```python
from build123d import *

# Parameters (mm, degrees)
SKETCH1_R           = 20
BOSS_EXTRUDE1_DEPTH = 10
SKETCH2_R           = 25
BOSS_EXTRUDE2_DEPTH = 60
FILLET1_R           = 25
SKETCH3_W           = 23.240720894
SKETCH3_H           = 7.34315937
BOSS_EXTRUDE3_DEPTH = 120
SKETCH4_R           = 7.943437771
BOSS_EXTRUDE4_DEPTH = 60
FILLET2_R           = 7
FILLET3_R           = 7
FILLET4_SIZE        = 10
FILLET4_SIZE_2      = 13


with BuildPart() as part:
    # Sketch1 → Boss-Extrude1 (new body)
    with BuildSketch(Plane(origin=(0, 0, 0), x_dir=(0, 0, -1), z_dir=(1, 0, 0))):
        Circle(SKETCH1_R)
    extrude(amount=BOSS_EXTRUDE1_DEPTH)

    # Sketch2 → Boss-Extrude2 (add)
    with BuildSketch(Plane(origin=(10, 0, 0), x_dir=(0, 0, -1), z_dir=(1, 0, 0))):
        Circle(SKETCH2_R)
    extrude(amount=BOSS_EXTRUDE2_DEPTH)

    # Fillet1
    fillet1_edges = [part.edges().sort_by_distance(p)[0] for p in [
        (70, 0, 25),
    ]]
    fillet(fillet1_edges, radius=FILLET1_R)

    # Sketch3 → Boss-Extrude3 (add)
    with BuildSketch(Plane.ZY):
        Rectangle(SKETCH3_W, SKETCH3_H)
    extrude(amount=-BOSS_EXTRUDE3_DEPTH)

    # Sketch4 → Boss-Extrude4 (add, symmetric)
    with BuildSketch(Plane(origin=(0, 3.671579685, 0), x_dir=(1, 0, 0), z_dir=(0, 1, 0))):
        with Locations(Location((103.030776269, 0, 0), (0, 0, 270))):
            Circle(SKETCH4_R)
    extrude(amount=BOSS_EXTRUDE4_DEPTH, both=True)

    # Fillet2
    fillet2_edges = [part.edges().sort_by_distance(p)[0] for p in [
        (103.030776269, 63.671579685, -7.943437771),
    ]]
    fillet(fillet2_edges, radius=FILLET2_R)

    # Fillet3
    fillet3_edges = [part.edges().sort_by_distance(p)[0] for p in [
        (103.030776269, -56.328420315, -7.943437771),
    ]]
    fillet(fillet3_edges, radius=FILLET3_R)

    # Fillet4
    # an asymmetric fillet: 13, 10 mm, written as the material it takes off along each edge
    with BuildSketch(Plane(origin=(120, -36.171579685, -11.620360447), x_dir=(-1, 0, 0), z_dir=(0, 1, 0)), Plane(origin=(120, 36.171579685, 11.620360447), x_dir=(-1, 0, 0), z_dir=(0, -1, 0))) as fillet4_piece_1:
        with BuildLine():
            Bezier((FILLET4_SIZE, 0), (0, 0), (0, FILLET4_SIZE_2), weights=[1, 0.707106781, 1])
            Line((0, FILLET4_SIZE_2), (0, 0))
            Line((0, 0), (FILLET4_SIZE, 0))
        make_face()
    extrude(amount=72.34315937, mode=Mode.SUBTRACT)


solid = part.part
```
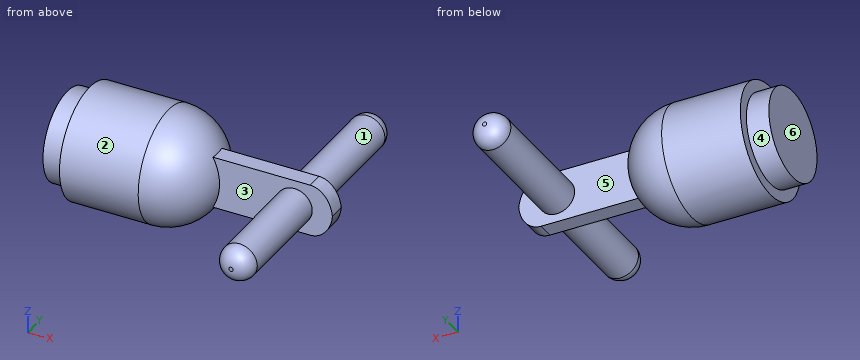
Design review of the part built by this model. Coordinates are the model's own, in mm. Face numbers are marked on the shaded views. A direction names the side the tool comes from. Round coordinates to 2 decimals unless told otherwise and drop trailing zeros. Write each loop counter-clockwise with the first axis right and the second up, starting at its lowest first coordinate (ties: lowest second). Pieces come first, ordered by that corner, then holes.
Item 1: For probe 1 along Y at (x, z) = (83.5, 4.5); probe 2 along Z at (x, y) = (95, -2); probe 3 along Z at (x, y) = (97, -11.5), list the stretches that pass through material, from the lowest coordinate up.
Item 2: We need section D-D on y = -35. Write out the cut boundary in (x, z), and give its area (3 significant figures).
Item 3: We need section C-C on x = 33. Write out the cut boundary in (y, z).
Item 4: The part is to be moulded in two halves that separate along X. For the marked faces 4, 5 and 6, say which applies: +X half, -X half, draft (parallel to the pull), parting line (faces both ways), or undercut.
Item 5: We need section A-A on y = -16. Write out the cut boundary in (x, z).
Item 6: For the marked faces 1, 2 and 3, list the 3-axis set-ups (+Z, -Z, +X, -X, +Y, -Y) from which the entire face can be reached by the end or side of a thin tool; tool diameter is ignored.
Item 7: We need section B-B on z = 17.5. Write out the cut boundary in (x, y), and give its area (3 significant figures).
Item 8: Clearance check with flat-ended pins moving along their axes: pin 1 Ø10 at (y, z) = (18.5, -19) entering from -X; pin 2 Ø3 at (x, z) = (37, 16) entering from -Y; pin 3 Ø3 at (y, z) = (-28.5, -1) entering from +X. State where each tip first meets the part, or that it passes through.
Returned:
1. probe 1: y = -3.67 to 3.67
1. probe 2: z = -11.62 to 11.62
1. probe 3: z = -5.17 to 5.17
2. outline: circle Ø15.89 at (103.03, 0)
2. area: 198 mm2
3. outline: circle Ø50 at (0, 0)
4. face 4: draft
4. face 5: undercut
4. face 6: -X half
5. outline: (0, -12) - (10, -12) - (10, -19.21) - (45, -19.21) arc R19.21 ccw to (45, 19.21) - (10, 19.21) - (10, 12) - (0, 12) - close; circle Ø15.89 at (103.03, 0)
6. face 1: +Y
6. face 2: -X
6. face 3: -Y
7. outline: (0, -9.68) - (10, -9.68) - (10, -17.85) - (45, -17.85) arc R17.85 ccw to (45, 17.85) - (10, 17.85) - (10, 9.68) - (0, 9.68) - close
7. area: 1,940 mm2
8. pin 1: stops at x = 10
8. pin 2: stops at y = -20.37
8. pin 3: stops at x = 110.97
